from build123d import *

# Parameters (mm, degrees)
BASE_PLATE_DEPTH                = 3
RAIN_PLATE_WEDGE_DEPTH          = 44
RAIN_PLATE_POCKET_DEPTH         = 20.8
SKETCH4_W                       = 33
SKETCH4_H                       = 12
LM393_BOARD_POCKET_DEPTH        = 9.5
RAIN_PLATE_PIN_HOLE_DEPTH       = 15
SKETCH6_W                       = 25
SKETCH6_H                       = 36
SKETCH6_W_2                     = 21
SKETCH6_H_2                     = 32
DHT11_SCREEN_WALLS_DEPTH        = 40
SKETCH7_W                       = 25
SKETCH7_H                       = 36
DHT11_SCREEN_ROOF_DEPTH         = 5
SKETCH8_W                       = 16.8
SKETCH8_H                       = 34
LDR_MODULE_POCKET_DEPTH         = 1.75
SKETCH9_R                       = 2
SKETCH9_R_2                     = 4
LDR_AND_SCREEN_WIRE_HOLES_DEPTH = 1.5
SKETCH10_R                      = 4
DHT11_WIRE_HOLE_DEPTH           = 2
SKETCH11_R                      = 1
FILAMENT_PIN_HOLES_DEPTH        = 1.55
SKETCH12_W                      = 3
SKETCH12_H                      = 22
LOUVRES_BACK_DEPTH              = 2
SKETCH13_W                      = 17
SKETCH13_H                      = 3
LOUVRES_STBD_DEPTH              = 2
SKETCH14_W                      = 17
SKETCH14_H                      = 3
LOUVRES_PORT_DEPTH              = 2


with BuildPart() as part:
    # Sketch1 → Base_plate (new body)
    with BuildSketch(Plane.XY.offset(373.2)):
        with BuildLine():
            Line((-131, -35), (-52, -35))
            ThreePointArc((-52, -35), (-49.171572875, -33.828427125), (-48, -31))
            Line((-48, -31), (-48, 31))
            ThreePointArc((-48, 31), (-49.171572875, 33.828427125), (-52, 35))
            Line((-52, 35), (-131, 35))
            ThreePointArc((-131, 35), (-133.828427125, 33.828427125), (-135, 31))
            Line((-135, 31), (-135, -31))
            ThreePointArc((-135, -31), (-133.828427125, -33.828427125), (-131, -35))
        make_face()
    extrude(amount=BASE_PLATE_DEPTH)

    # Sketch2 → Rain_plate_wedge (add)
    with BuildSketch(Plane(origin=(-104, 0, 0), x_dir=(0, 0, -1), z_dir=(1, 0, 0))):
        Polygon((-376.19, -27), (-376.19, 26), (-406.444863729, 26), (-377, -25), (-377, -27), align=None)
    extrude(amount=RAIN_PLATE_WEDGE_DEPTH)

    # Sketch3 → Rain_plate_pocket (cut, symmetric)
    with BuildSketch(Plane(origin=(-82, 0, 0), x_dir=(0, 0, -1), z_dir=(1, 0, 0))):
        Polygon((-377.859807621, -24.110769515), (-405.859807621, 24.386653096), (-403.694744112, 25.636653096), (-375.694744112, -22.860769515), align=None)
    extrude(amount=RAIN_PLATE_POCKET_DEPTH, both=True, mode=Mode.SUBTRACT)

    # Sketch4 → LM393_board_pocket (cut, symmetric)
    with BuildSketch(Plane(origin=(0, 17.5, 0), x_dir=(1, 0, 0), z_dir=(0, 1, 0))):
        with Locations((-82, -384.2)):
            Rectangle(SKETCH4_W, SKETCH4_H)
    extrude(amount=LM393_BOARD_POCKET_DEPTH, both=True, mode=Mode.SUBTRACT)

    # Sketch5 → Rain_plate_pin_hole (cut, symmetric)
    with BuildSketch(Plane.XY.offset(404.7)):
        with BuildLine():
            Line((-85, 16), (-79, 16))
            ThreePointArc((-79, 16), (-77.585786438, 16.585786438), (-77, 18))
            Line((-77, 18), (-77, 22))
            ThreePointArc((-77, 22), (-77.585786438, 23.414213562), (-79, 24))
            Line((-79, 24), (-85, 24))
            ThreePointArc((-85, 24), (-86.414213562, 23.414213562), (-87, 22))
            Line((-87, 22), (-87, 18))
            ThreePointArc((-87, 18), (-86.414213562, 16.585786438), (-85, 16))
        make_face()
    extrude(amount=RAIN_PLATE_PIN_HOLE_DEPTH, both=True, mode=Mode.SUBTRACT)

    # Sketch6 → DHT11_screen_walls (add)
    with BuildSketch(Plane.XY.offset(376.2)):
        with Locations((-120.5, 0)):
            Rectangle(SKETCH6_W, SKETCH6_H)
        with Locations((-120.5, 0)):
            Rectangle(SKETCH6_W_2, SKETCH6_H_2, mode=Mode.SUBTRACT)
    extrude(amount=DHT11_SCREEN_WALLS_DEPTH)

    # Sketch7 → DHT11_screen_roof (add)
    with BuildSketch(Plane.XY.offset(416.2)):
        with Locations((-120.5, 0)):
            Rectangle(SKETCH7_W, SKETCH7_H)
    extrude(amount=DHT11_SCREEN_ROOF_DEPTH)

    # Sketch8 → LDR_module_pocket (cut, symmetric)
    with BuildSketch(Plane.XY.offset(419.95)):
        with Locations((-121, 0)):
            Rectangle(SKETCH8_W, SKETCH8_H)
    extrude(amount=LDR_MODULE_POCKET_DEPTH, both=True, mode=Mode.SUBTRACT)

    # Sketch9 → LDR_and_screen_wire_holes (cut, symmetric)
    with BuildSketch(Plane.XY.offset(417.2)):
        with Locations((-121, -14)):
            Circle(SKETCH9_R)
        with Locations((-121, 0)):
            Circle(SKETCH9_R_2)
    extrude(amount=LDR_AND_SCREEN_WIRE_HOLES_DEPTH, both=True, mode=Mode.SUBTRACT)

    # Sketch10 → DHT11_wire_hole (cut, symmetric)
    with BuildSketch(Plane.XY.offset(374.7)):
        with Locations((-121, 0)):
            Circle(SKETCH10_R)
    extrude(amount=DHT11_WIRE_HOLE_DEPTH, both=True, mode=Mode.SUBTRACT)

    # Sketch11 → Filament_pin_holes (cut, symmetric)
    with BuildSketch(Plane.XY.offset(374.25)):
        with Locations((-90, 20)):
            Circle(SKETCH11_R)
        with Locations((-90, -20)):
            Circle(SKETCH11_R)
    extrude(amount=FILAMENT_PIN_HOLES_DEPTH, both=True, mode=Mode.SUBTRACT)

    # Sketch12 → Louvres_back (cut, symmetric)
    with BuildSketch(Plane(origin=(-132, 0, 0), x_dir=(0, 0, -1), z_dir=(1, 0, 0))):
        with Locations((-383.7, 0)):
            Rectangle(SKETCH12_W, SKETCH12_H)
        with Locations((-390.2, 0)):
            Rectangle(SKETCH12_W, SKETCH12_H)
        with Locations((-396.7, 0)):
            Rectangle(SKETCH12_W, SKETCH12_H)
        with Locations((-403.2, 0)):
            Rectangle(SKETCH12_W, SKETCH12_H)
        with Locations((-409.7, 0)):
            Rectangle(SKETCH12_W, SKETCH12_H)
    extrude(amount=LOUVRES_BACK_DEPTH, both=True, mode=Mode.SUBTRACT)

    # Sketch13 → Louvres_stbd (cut, symmetric)
    with BuildSketch(Plane(origin=(0, 17, 0), x_dir=(1, 0, 0), z_dir=(0, 1, 0))):
        with Locations((-120.5, -383.7)):
            Rectangle(SKETCH13_W, SKETCH13_H)
        with Locations((-120.5, -390.2)):
            Rectangle(SKETCH13_W, SKETCH13_H)
        with Locations((-120.5, -396.7)):
            Rectangle(SKETCH13_W, SKETCH13_H)
        with Locations((-120.5, -403.2)):
            Rectangle(SKETCH13_W, SKETCH13_H)
        with Locations((-120.5, -409.7)):
            Rectangle(SKETCH13_W, SKETCH13_H)
    extrude(amount=LOUVRES_STBD_DEPTH, both=True, mode=Mode.SUBTRACT)

    # Sketch14 → Louvres_port (cut, symmetric)
    with BuildSketch(Plane(origin=(0, -17, 0), x_dir=(1, 0, 0), z_dir=(0, 1, 0))):
        with Locations((-120.5, -383.7)):
            Rectangle(SKETCH14_W, SKETCH14_H)
        with Locations((-120.5, -390.2)):
            Rectangle(SKETCH14_W, SKETCH14_H)
        with Locations((-120.5, -396.7)):
            Rectangle(SKETCH14_W, SKETCH14_H)
        with Locations((-120.5, -403.2)):
            Rectangle(SKETCH14_W, SKETCH14_H)
        with Locations((-120.5, -409.7)):
            Rectangle(SKETCH14_W, SKETCH14_H)
    extrude(amount=LOUVRES_PORT_DEPTH, both=True, mode=Mode.SUBTRACT)


solid = part.part
Here's how the part is built. I have some questions about the finished solid (model axes, mm). A direction names the side the tool comes from. Give positions to 0.01 mm unless a question says otherwise; leave off trailing zeros. Loops run counter-clockwise (first coordinate to the right, second up) from the corner with the lowest first, then second, coordinate; pieces in that order, holes last. Notation, with made-up numbers: (66.25, 11.25) -> (124.25, 11.25) arc R28 cw to (124.25, 30.25) -> close; hole circle Ø5 at (0, 13.5). An arc over 180 degrees is marked (long way). Answer as a JSON object with one key per item and string values. Group by question number.
Item 1: Imagine slicing it at D-D on x = -73.5. Write out the boundary of the cut face in (y, z).
Item 2: Imagine slicing it at A-A on x = -86. Write out the boundary of the cut face in (y, z).
Item 3: Will these pins go through, and if not, where does the flat tip stop? pin 1 (1 mm diameter, centred on y = -15, z = 402, fed in from +X); pin 2 (12 mm diameter, centred on x = -64, z = 393, fed in from -Y); pin 3 (1 mm diameter, centred on y = -16.5, z = 397, fed in from -X).
Item 4: On a 3-axis mill with a long thin cutter (end or side, diameter ignored), from which of +Z, -Z, +X, -X, +Y, -Y can I reach the whole of each face in a straight line? I mean faces 1 (the flat face through (-132, 0, 404.7)), 2 (the cylindrical face through (-77.6, 16.57, 394.81)), 3 (the flat face through (-112, 17, 403)). Say none if no direction works.
Item 5: Imagine slicing it at C-C on y = -15. Write out the boundary of the cut face in (x, z).
Item 6: Thinking about a two-plate mould opening in Y: for faces 4 (the flat face through (-90, 20, 375.8)), 5 (the cylindrical face through (-133.797, 33.859, 374.679)), 6 (the flat face through (-104, 12, 385)), which applies, pulls with the +Y half, pulls with the -Y half, needs draft (parallel to the pull), parting line crosses it, or undercut?
Item 7: Imagine slicing it at B-B on z = 414.5. Write out the boundary of the cut face in (x, y), then the cut area to 3 significant figures.
Item 8: I need wall thicknesses on L1, parallel to X at y = 7.5, z = 377.5; L2, parallel to Y at x = -90, z = 375.1; L3, parallel to Y at x = -121, z = 416.7. Which ranges of each line are inside material? Lowest first, please.
Answer list:
{
 "1": {"outline": "(-35, 373.2) -> (35, 373.2) -> (35, 376.2) -> (26, 376.2) -> (26, 378.2) -> (8, 378.2) -> (8, 390.2) -> (26, 390.2) -> (26, 406.44) -> (24.54, 405.6) -> (25.64, 403.69) -> (-22.86, 375.69) -> (-23.96, 377.6) -> (-25, 377) -> (-27, 377) -> (-27, 376.2) -> (-35, 376.2) -> close"},
 "2": {"outline": "(-35, 373.2) -> (35, 373.2) -> (35, 376.2) -> (26, 376.2) -> (26, 378.2) -> (8, 378.2) -> (8, 390.2) -> (16.27, 390.2) -> (16.27, 398.29) -> (-22.86, 375.69) -> (-23.96, 377.6) -> (-25, 377) -> (-27, 377) -> (-27, 376.2) -> (-35, 376.2) -> close; (23.73, 390.2) -> (26, 390.2) -> (26, 406.44) -> (24.54, 405.6) -> (25.64, 403.69) -> (23.73, 402.6) -> close"},
 "3": {"pin 1": "stops at x = -108", "pin 2": "stops at y = -6.48", "pin 3": "stops at x = -133"},
 "4": {"face 1": "-X", "face 2": "+Z", "face 3": "+Y, -Y"},
 "5": {"outline": "(-135, 373.2) -> (-48, 373.2) -> (-48, 376.2) -> (-60, 376.2) -> (-60, 382.77) -> (-61.2, 382.77) -> (-61.2, 380.23) -> (-102.8, 380.23) -> (-102.8, 382.77) -> (-104, 382.77) -> (-104, 376.2) -> (-108, 376.2) -> (-108, 421.2) -> (-112.6, 421.2) -> (-112.6, 418.2) -> (-119.27, 418.2) -> (-119.27, 416.2) -> (-110, 416.2) -> (-110, 376.2) -> (-131, 376.2) -> (-131, 416.2) -> (-122.73, 416.2) -> (-122.73, 418.2) -> (-129.4, 418.2) -> (-129.4, 421.2) -> (-133, 421.2) -> (-133, 376.2) -> (-135, 376.2) -> close"},
 "6": {"face 4": "undercut", "face 5": "pulls with the +Y half", "face 6": "needs draft"},
 "7": {"outline": "(-133, -18) -> (-108, -18) -> (-108, 18) -> (-133, 18) -> close; hole (-131, -16) -> (-110, -16) -> (-110, 16) -> (-131, 16) -> close", "area": "228 mm2"},
 "8": {"L1": "x = -133 to -131, -110 to -108, -104 to -60", "L2": "y = -35 to -21, -19 to 19, 21 to 35", "L3": "y = -18 to -16, -12 to -4, 4 to 18"}
}
